Source: three-view drawing plus pictorial views. Frame: mm from the lowest corner of the part. Coordinates: 2 decimals unless noted, no trailing zeros. Loops run counter-clockwise (first coordinate to the right, second up) from the corner with the lowest first, then second, coordinate; pieces in that order, holes last. Notation, with made-up numbers: M 44.25,39.5 L 84.25,39.5 A7 ccw 84.25,50.5 Z; hole C 12,-22 d3. An arc over 180 degrees is marked long. Write each question's results on one line, items separated by ' | '. Start each with the question number.
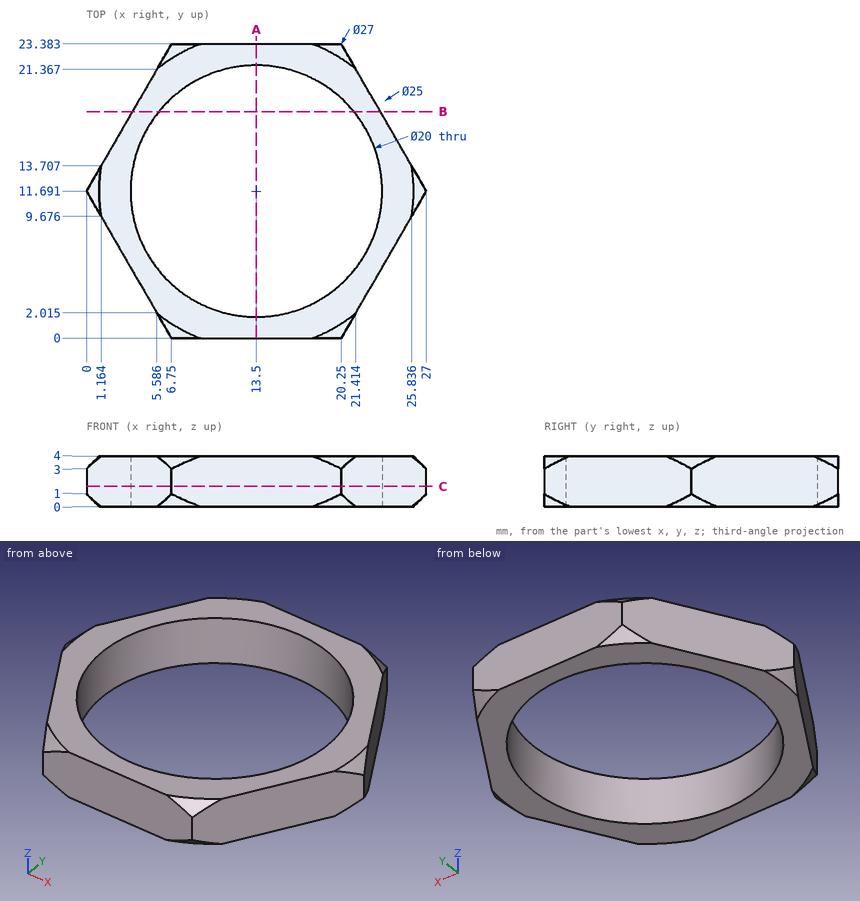
Item 1: Contact query for flat-ended pins moving along their axis: P1, Ø1.5, axis at x = 4.5, z = 0.5, coming from the +Y side (1 decimal); P2, Ø12, axis at x = 6.5, y = 14, coming from the -Z side. Output: stop coordinate, or through.
Item 2: Section B-B, the plane y = 18. Return loops of the section in (x, z), plus the area to 3 significant figures.
Item 3: Section A-A, the plane x = 13.5. Return loops of the section in (y, z).
Item 4: Section C-C, the plane z = 1.6. Return loops of the section in (x, y), plus the area to 3 significant figures.
Item 5: Ray query, L1, parallel to Y at x = 13.5, z = 1.2; L2, parallel to Y at x = 14.5, z = 3.75; L3, parallel to X at y = 6.5, z = 3.05 (1 decimal). Return the intervals inside material, ascending. Write a range as [from, to].
Solutions:
1) P1: stops at y = 20.8 | P2: stops at z = 0
2) outline: M 3.64,0 L 5.74,0 L 5.74,4 L 3.64,4 Z; M 21.26,0 L 23.36,0 L 23.36,4 L 21.26,4 Z | area: 16.8 mm²
3) outline: M 0,0 L 1.69,0 L 1.69,4 L 0,4 Z; M 21.69,0 L 23.38,0 L 23.38,4 L 21.69,4 Z
4) outline: M 0,11.69 L 6.75,0 L 20.25,0 L 27,11.69 L 20.25,23.38 L 6.75,23.38 Z; hole C 13.5,11.69 d20 | area: 159 mm²
5) L1: y = [0, 1.69], [21.69, 23.38] | L2: y = [0, 1.74], [21.64, 23.38] | L3: x = [3, 5], [22, 24]
